CAD build for the part. Positions are in the model's coordinates, mm. A direction names the side the tool comes from. Give positions to 0.01 mm unless a question says otherwise; leave off trailing zeros. Write each loop counter-clockwise with the first axis right and the second up, starting at its lowest first coordinate (ties: lowest second). Pieces come first, ordered by that corner, then holes. Notation, with made-up numbers: (-24, 2) -> (-1, 2) arc R14 ccw to (-1, 27) -> close; hole circle Ø4 at (-28.5, -27). An arc over 180 degrees is marked (long way). Use one line per item in the form item = value. Start each with the question number.
from build123d import *

# Parameters (mm, degrees)
BOSS_EXTRUDE1_DEPTH     = 78
CUT_EXTRUDE1_DEPTH      = 98.015462685
CUT_EXTRUDE1_DEPTH_BACK = 98.015462685
CUT_EXTRUDE2_DEPTH      = 98.015462685
CUT_EXTRUDE2_DEPTH_BACK = 10
SKETCH3_R               = 4
CHAMFER1_SIZE           = 1.5


with BuildPart() as part:
    # Sketch1 → Boss-Extrude1 (new body)
    with BuildSketch(Plane(origin=(0, 0, 0), x_dir=(0, 0, -1), z_dir=(1, 0, 0))):
        with BuildLine():
            Line((0, 8), (3.75, 5.834936491))
            ThreePointArc((3.75, 5.834936491), (5.25, 5.834936491), (6, 7.133974596))
            Line((6, 7.133974596), (6, 32))
            Line((6, 32), (24, 32))
            Line((24, 32), (24, 25))
            Line((24, 25), (25.787630389, 26.5))
            Line((25.787630389, 26.5), (27.787630389, 26.5))
            Line((27.787630389, 26.5), (29.575260778, 25))
            Line((29.575260778, 25), (46.5, 25))
            Line((46.5, 25), (48, 23.5))
            Line((48, 23.5), (48, 12.166666667))
            ThreePointArc((48, 12.166666667), (47.560660172, 11.106006495), (46.5, 10.666666667))
            Line((46.5, 10.666666667), (20.7, 10.666666667))
            ThreePointArc((20.7, 10.666666667), (19.639339828, 10.227326838), (19.2, 9.166666667))
            Line((19.2, 9.166666667), (19.2, 1.5))
            ThreePointArc((19.2, 1.5), (18.760660172, 0.439339828), (17.7, 0))
            Line((17.7, 0), (1.5, 0))
            ThreePointArc((1.5, 0), (0.439339828, 0.439339828), (0, 1.5))
            Line((0, 1.5), (0, 8))
        make_face()
    extrude(amount=BOSS_EXTRUDE1_DEPTH)

    # Sketch2 → Cut-Extrude1 (cut, two sides: drawn at the far end of the back side and taken through both)
    with BuildSketch(Plane.XY.offset(-CUT_EXTRUDE1_DEPTH_BACK)):
        Polygon((3.561829482, 32), (3.561829482, 21.333333333), (0, 13.333333333), (0, 32), align=None)
        Polygon((78, 13.333333333), (74.438170518, 21.333333333), (74.438170518, 32), (78, 32), align=None)
    extrude(amount=CUT_EXTRUDE1_DEPTH + CUT_EXTRUDE1_DEPTH_BACK, mode=Mode.SUBTRACT)

    # Sketch3 → Cut-Extrude2 (cut, two sides: drawn at the far end of the back side and taken through both)
    with BuildSketch(Plane(origin=(0, 32, 0), x_dir=(1, 0, 0), z_dir=(0, 1, 0)).offset(-CUT_EXTRUDE2_DEPTH_BACK)):
        with Locations(Location((15.561829482, 15, 0), (0, 0, 270))):
            Circle(SKETCH3_R)
        with Locations(Location((62.438170518, 15, 0), (0, 0, 270))):
            Circle(SKETCH3_R)
        with Locations(Location((39, 15, 0), (0, 0, 270))):
            Circle(SKETCH3_R)
    extrude(amount=CUT_EXTRUDE2_DEPTH + CUT_EXTRUDE2_DEPTH_BACK, mode=Mode.SUBTRACT)

    # Chamfer1
    chamfer1_edges = [part.edges().sort_by_distance(p)[0] for p in [
        (15.561829482, 32, -19),
        (62.438170518, 32, -19),
        (39, 32, -19),
    ]]
    chamfer(chamfer1_edges, length=CHAMFER1_SIZE)


solid = part.part
1) Pin check, flat tips, straight feed: pin 1 (2 mm diameter, centred on x = 27.5, y = 29, fed in from -Z); pin 2 (4 mm diameter, centred on x = 63, z = -13, fed in from +Y); pin 3 (6.5 mm diameter, centred on x = 62.44, z = -15, fed in from +Y). Stop position of each tip, or through.
2) Cut at A-A (x = 45.5). Give the cut face in (y, z).
3) Cut at C-C (y = 19). Give the cut face in (x, z), and give its area (3 significant figures).
4) Two-plate mould, pull along Z, no slides. Class faces 1 (the face through (39, 22, -15)), 2 (the face through (16, 22, -15)), 3 (the face through (38.45, 10.24, -19.65)), 4 (the face through (3.562, 26, -23)): released by +Z, released by -Z, zero draft, split by the parting line, or undercut.
5) 3-axis set-ups, long thin cutter, end or side, ignore diameter. For faces 5 (the face through (13.128, 26.19, -18.174)), 6 (the face through (38, 5, -19.2)), 7 (the face through (74.438, 25, -23)), 8 (the face through (39, 25, -38)): which of +Z, -Z, +X, -X, +Y, -Y reach the whole face in a straight line?
6) Wall check: line 1 along X through (y, z) = (24.75, -15); line 2 along Z through (x, y) = (39, 27.25); line 3 along Z through (x, y) = (58, 16). Give the ranges that are in metal, low to high. Write a range as from..to.
7) Cut at B-B (z = -15). Give the cut face in (x, y), and give its area (3 significant figures).
Final values:
q1.pin_1 = -24
q1.pin_2 = 30.58
q1.pin_3 = 22
q2.outline = (0, -17.7) arc R1.5 ccw to (1.5, -19.2) -> (9.17, -19.2) arc R1.5 cw to (10.67, -20.7) -> (10.67, -46.5) arc R1.5 ccw to (12.17, -48) -> (23.5, -48) -> (25, -46.5) -> (25, -29.58) -> (26.5, -27.79) -> (26.5, -25.79) -> (25, -24) -> (32, -24) -> (32, -6) -> (7.13, -6) arc R1.5 cw to (5.83, -3.75) -> (8, 0) -> (1.5, 0) arc R1.5 ccw to (0, -1.5) -> close
q3.outline = (2.52, -48) -> (75.48, -48) -> (75.48, -6) -> (2.52, -6) -> close
q3.area = 3,060 mm^2
q4.face_1 = undercut
q4.face_2 = undercut
q4.face_3 = released by -Z
q4.face_4 = zero draft
q5.face_5 = +Y
q5.face_6 = -Z, +X, -X, -Y
q5.face_7 = +Z, -Z, +X, +Y
q5.face_8 = -Z, +X, -X, +Y
q6.line_1 = 3.56..11.56, 19.56..35, 43..58.44, 66.44..74.44
q6.line_2 = -24..-19, -11..-6
q6.line_3 = -48..-6
q7.outline = (0, 0) -> (78, 0) -> (78, 13.33) -> (74.44, 21.33) -> (74.44, 32) -> (67.94, 32) -> (66.44, 30.5) -> (66.44, 22) -> (58.44, 22) -> (58.44, 30.5) -> (56.94, 32) -> (44.5, 32) -> (43, 30.5) -> (43, 22) -> (35, 22) -> (35, 30.5) -> (33.5, 32) -> (21.06, 32) -> (19.56, 30.5) -> (19.56, 22) -> (11.56, 22) -> (11.56, 30.5) -> (10.06, 32) -> (3.56, 32) -> (3.56, 21.33) -> (0, 13.33) -> close
q7.area = 2,140 mm^2
